CAD build for the part. Positions are in the model's coordinates, mm. Face numbers are marked on the shaded views. A direction names the side the tool comes from. Round coordinates to 2 decimals unless told otherwise and drop trailing zeros. Loops run counter-clockwise (first coordinate to the right, second up) from the corner with the lowest first, then second, coordinate; pieces in that order, holes last. Notation, with made-up numbers: (-20.75, 9.25) -> (26.25, 9.25) arc R30 ccw to (26.25, 45.25) -> close; hole circle Ø11 at (16, 63). An arc over 180 degrees is marked (long way). Answer as CSV lines item,"result".
Solid Edge part; units mm, degrees
sketch "Sketch1" plane through (0, 0, 0) normal (0, 0, 1) x (1, 0, 0)
  line L0 (200, 0) -> (105, 0)
  arc A0 (105, 0) -> (0, 105) centre (0, 0) ccw
  line L1 (0, 105) -> (0, 242)
  line L2 (0, 242) -> (200, 242)
  line L3 (200, 242) -> (200, 0)
extrude "Protrusion1" add sketch "Sketch1" along normal blind 40
fillet "Redondeo_1" radius 4 5 edges at (200, 0, 20) (0, 105, 20) (105, 0, 20) (200, 242, 20) (0, 242, 20)
shell "Espesor_2" thickness 1.5 removed faces 1 at (168.6667, 42.7533, 0)
sketch "Sketch2" plane through (100, 121, 40) normal (0, 0, 1) x (1, 0, 0)
  arc A0 (-100, -3.2) -> (17.8, -121) centre (-100, -121) cw
  line L0 (17.8, -121) -> (19.8, -121)
  arc A1 (-100, -1.2) -> (19.8, -121) centre (-100, -121) cw
  line L1 (-100, -1.2) -> (-100, -3.2)
extrude "ProtrusiónExtruida_2" add sketch "Sketch2" along normal blind 0.01
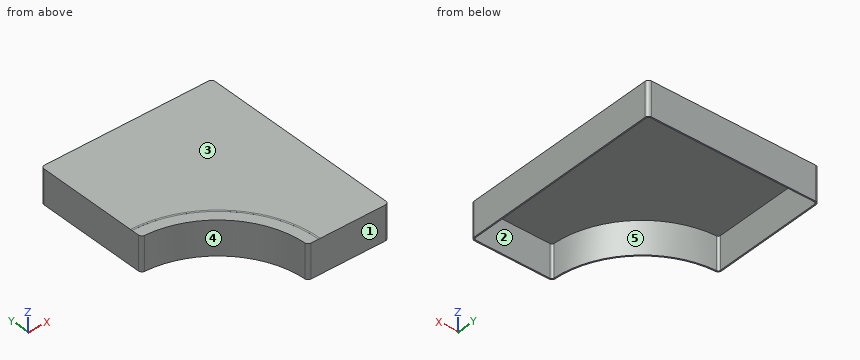
Q1. Two-plate mould, pull along X, no slides. Class the marked faces 3, 4 and 5: pulls with the +X half, pulls with the -X half, needs draft (parallel to the pull), parting line crosses it, or undercut.
Results:
face 3,"needs draft"
face 4,"pulls with the -X half"
face 5,"undercut"
Q2. Slice it at C-C, the plane y = 138. Give the cut face in (x, z), and give its area (4 significant figures).
Results:
outline,"(0, 0) -> (1.5, 0) -> (1.5, 38.5) -> (198.5, 38.5) -> (198.5, 0) -> (200, 0) -> (200, 40) -> (0, 40) -> close"
area,"415.5 mm2"
Q3. Slice it at B-B, the plane x = 177. Give the cut face in (y, z), and give its area (4 significant figures).
Results:
outline,"(0, 0) -> (1.5, 0) -> (1.5, 38.5) -> (240.5, 38.5) -> (240.5, 0) -> (242, 0) -> (242, 40) -> (0, 40) -> close"
area,"478.5 mm2"
Q4. Tool access for the marked faces 1 and 2: list every direction of +Z, -Z, +X, -X, +Y, -Y with a clear straight run to the whole face (end or side of a thin tool).
Results:
face 1,"+Z, -Z, +X, -X, -Y"
face 2,"-Z"
Q5. Slice it at A-A, the plane z = 17.5. Give the cut face in (x, y), and give its area (3 significant figures).
Results:
outline,"(0, 108.93) arc R4 ccw to (3.85, 104.93) arc R105 cw to (104.93, 3.85) arc R4 ccw to (108.93, 0) -> (196, 0) arc R4 ccw to (200, 4) -> (200, 238) arc R4 ccw to (196, 242) -> (4, 242) arc R4 ccw to (0, 238) -> close; hole (1.5, 108.93) arc R2.5 ccw to (3.91, 106.43) arc R106.5 cw to (106.43, 3.91) arc R2.5 ccw to (108.93, 1.5) -> (196, 1.5) arc R2.5 ccw to (198.5, 4) -> (198.5, 238) arc R2.5 ccw to (196, 240.5) -> (4, 240.5) arc R2.5 ccw to (1.5, 238) -> close"
area,"1,240 mm2"
Q6. Drop flat-ended pins along their axis: pin 1 Ø6 at (x, y) = (90.5, 135.5) entering from +Z; pin 2 Ø1 at (x, y) = (178, 185) entering from -Z. Give the stop position or say it passes through.
Results:
pin 1,"z = 40"
pin 2,"z = 38.5"
Q7. Probe L1, parallel to Y at x = 120, z = 34; L2, parallel to X at y = 139, z = 18.5; L3, parallel to Z at x = 125.5, y = 170. List the from-to ranges inside material, lowest first. Write a range as [from, to].
Results:
L1,"[0, 1.5], [240.5, 242]"
L2,"[0, 1.5], [198.5, 200]"
L3,"[38.5, 40]"
